Source: CAD feature listing. Evaluate the final solid. Frame: model axes, mm. A direction names the side the tool comes from. Coordinates: 2 decimals unless noted, no trailing zeros. Write each loop counter-clockwise with the first axis right and the second up, starting at its lowest first coordinate (ties: lowest second). Pieces come first, ordered by that corner, then holes. Notation, with made-up numbers: M 39,-28.75 L 95,-28.75 A31 cw 95,9.25 Z; hole C -29.5,2 d9. An arc over 180 degrees is marked long. Write item = value, one per line. Start each with the question number.
1. Line query: line 1 along Z through (x, y) = (15, 0.65); line 2 along X through (y, z) = (5.75, 8.75); line 3 along Z through (x, y) = (1.75, 5). Output: solid intervals per line, ascending.
2. Access query for faces 1 (the face through (12.86, 5.03, 0.81)), 2 (the face through (0, 3, 6)). Directions: +Z, -Z, +X, -X, +Y, -Y. A direction counts if a zero-diameter tool reaches every point of the face in a straight line with its end or side. Return the directions, or none.
3. Section query B-B (x = 15). Output: boundary loops of the cut face in (y, z), then the cut area to 3 significant figures.
4. Pin query (flat end, axial travel): pin 1 Ø0.9 at (x, z) = (1.5, 6) entering from +Y; pin 2 Ø2.5 at (x, z) = (1.5, 6) entering from +Y. Return the tip coordinate at first contact, or that it passes through.
5. Pull-direction query (Z, two-part tool) for faces 3 (the face through (10, 3, 0)), 4 (the face through (7.4, 1.6, 9.5)), 5 (the face through (19, 6.8, 9)); classes: pulls with the +Z half, pulls with the -Z half, needs draft (parallel to the pull), parting line crosses it, or undercut.
6. Section query A-A (y = 3.75). Output: boundary loops of the cut face in (x, z).
7. Section query C-C (z = 9). Output: boundary loops of the cut face in (x, y), then the cut area to 3 significant figures.
8. Section query D-D (x = 12.75). Output: boundary loops of the cut face in (y, z).
```python
from build123d import *

# Parameters (mm, degrees)
SKETCH_1_W          = 20
SKETCH_1_H          = 12
SKETCH_1_R          = 2.1
SKETCH_1_R_2        = 0.6
EXTRUDE_1_DEPTH     = 3.3
EXTRUDE_START       = 3.3
EXTRUDE_4_DEPTH     = 3.5
SKETCH_2_R          = 0.75
CUT_EXTRUDE_1_DEPTH = 29.930952283
CUT_EXTRUDE_START   = 24
SKETCH_2_4_R        = 1
CUT_EXTRUDE_2_DEPTH = 5.8
SKETCH_3_R          = 0.35
CUT_EXTRUDE_3_DEPTH = 25.294855422


with BuildPart() as part:
    # 草图1 → 凸台-拉伸1 (new body)
    with BuildSketch(Plane(origin=(0, 0, 0), x_dir=(1, 0, 0), z_dir=(0, 1, 0))):
        with Locations((10, -6)):
            Rectangle(SKETCH_1_W, SKETCH_1_H)
        with BuildLine():
            ThreePointArc((12.439835428, -3.613463312), (18.220575086, -7.370363498), (11.50515478, -5.81011348))
            ThreePointArc((11.50515478, -5.81011348), (7.454652656, -2.789434091), (12.439835428, -3.613463312))
        make_face(mode=Mode.SUBTRACT)
        with Locations(Location((5, -6, 0), (0, 0, 270))):
            Circle(SKETCH_1_R, mode=Mode.SUBTRACT)
        with Locations(Location((7.678736094, -8.970584613, 0), (0, 0, 270))):
            Circle(SKETCH_1_R_2, mode=Mode.SUBTRACT)
    extrude(amount=EXTRUDE_1_DEPTH)

    # 草图1<6> → 凸台-拉伸4 (add)
    with BuildSketch(Plane(origin=(0, 0, 0), x_dir=(1, 0, 0), z_dir=(0, 1, 0)).offset(EXTRUDE_START)):
        with BuildLine():
            Line((7.958677072, 0), (0, 0))
            Line((0, 0), (0, -12))
            Line((0, -12), (5.925840657, -12))
            ThreePointArc((5.925840657, -12), (4.429268792, -10.270954659), (4.319841502, -7.986802561))
            ThreePointArc((4.319841502, -7.986802561), (3.000111311, -5.359340003), (5.600909971, -3.987810345))
            ThreePointArc((5.600909971, -3.987810345), (6.188678117, -1.644412009), (7.958677072, 0))
        make_face()
        with BuildLine():
            Line((20, 0), (11.735482653, 0))
            ThreePointArc((11.735482653, 0), (12.869036074, -0.819060885), (13.675372646, -1.961700559))
            ThreePointArc((13.675372646, -1.961700559), (18.910698319, -7.664012819), (11.171707216, -7.845717845))
            ThreePointArc((11.171707216, -7.845717845), (11.090844977, -7.871351024), (11.009487245, -7.895365208))
            ThreePointArc((11.009487245, -7.895365208), (10.945672327, -10.226422042), (9.43163153, -12))
            Line((9.43163153, -12), (20, -12))
            Line((20, -12), (20, 0))
        make_face()
    extrude(amount=EXTRUDE_4_DEPTH)

    # 草图2 → 切除-拉伸1 (cut, through all)
    with BuildSketch(Plane(origin=(5, -17.2, 6), x_dir=(0, 0, -1), z_dir=(0, 1, 0))):
        with Locations(Location((0, 3.5, 0), (0, 0, 180))):
            Circle(SKETCH_2_R)
        with Locations(Location((-4.7, -10, 0), (0, 0, 49.37814182))):
            Circle(SKETCH_2_R)
        with Locations(Location((4.7, -10, 0), (0, 0, 229.37814182))):
            Circle(SKETCH_2_R)
    extrude(amount=CUT_EXTRUDE_1_DEPTH, mode=Mode.SUBTRACT)

    # 草图2<4> → 切除-拉伸2 (cut)
    with BuildSketch(Plane(origin=(5, -17.2, 6), x_dir=(0, 0, -1), z_dir=(0, 1, 0)).offset(CUT_EXTRUDE_START)):
        with Locations(Location((0, 3.5, 0), (0, 0, 180))):
            Circle(SKETCH_2_4_R)
        with Locations(Location((-4.7, -10, 0), (0, 0, 180))):
            Circle(SKETCH_2_4_R)
        with Locations(Location((4.7, -10, 0), (0, 0, 180))):
            Circle(SKETCH_2_4_R)
    extrude(amount=-CUT_EXTRUDE_2_DEPTH, mode=Mode.SUBTRACT)

    # 草图3 → 切除-拉伸3 (cut, through all)
    with BuildSketch(Plane(origin=(0, 0, 0), x_dir=(1, 0, 0), z_dir=(0, 1, 0))):
        with Locations(Location((1.5, -1.5, 0), (0, 0, 270))):
            Circle(SKETCH_3_R)
        with Locations(Location((1.5, -10.5, 0), (0, 0, 270))):
            Circle(SKETCH_3_R)
        with Locations(Location((18.5, -10.5, 0), (0, 0, 270))):
            Circle(SKETCH_3_R)
        with Locations(Location((18.5, -1.5, 0), (0, 0, 270))):
            Circle(SKETCH_3_R)
    extrude(amount=CUT_EXTRUDE_3_DEPTH, mode=Mode.SUBTRACT)


solid = part.part
```
Results are:
q1.line_1 = 0 to 0.55, 2.05 to 2.5, 9.5 to 9.95, 11.45 to 12
q1.line_2 = 0 to 4.19, 11.17 to 11.76, 18.24 to 20
q1.line_3 = 0 to 1.26, 1.74 to 5.03, 6.97 to 10.26, 10.74 to 12
q2.face_1 = +Y
q2.face_2 = +Z, -Z, -X, +Y, -Y
q3.outline = M 0,0 L 6.8,0 L 6.8,0.3 L 1,0.3 L 1,0.55 L 0,0.55 Z; M 0,2.05 L 1,2.05 L 1,2.3 L 3.3,2.3 L 3.3,2.5 L 0,2.5 Z; M 0,9.5 L 3.3,9.5 L 3.3,9.7 L 1,9.7 L 1,9.95 L 0,9.95 Z; M 0,11.45 L 1,11.45 L 1,11.7 L 6.8,11.7 L 6.8,12 L 0,12 Z
q3.area = 6.40 mm^2
q4.pin_1 = through
q4.pin_2 = 6.8
q5.face_3 = pulls with the -Z half
q5.face_4 = undercut
q5.face_5 = needs draft
q6.outline = M 0,0 L 7.96,0 A4.25 cw 5.6,3.99 A2.1 cw 4.32,7.99 A3.5 cw 5.93,12 L 0,12 Z; M 9.43,12 A3.5 cw 11.01,7.9 A4.25 cw 11.17,7.85 A4.25 cw 14.16,10.17 A1 cw long 15.84,10.17 A4.25 cw 15.84,1.83 A1 cw long 14.16,1.83 A4.25 cw 13.68,1.96 A4.25 cw 11.74,0 L 20,0 L 20,12 Z; hole C 1.5,6 d2; hole C 1.5,1.5 d0.7; hole C 1.5,10.5 d0.7; hole C 18.5,1.5 d0.7; hole C 18.5,10.5 d0.7
q7.outline = M 0,0 L 7.08,0 L 7.08,3.3 L 4.18,3.3 L 4.18,6.8 L 0,6.8 Z; M 8.28,0 L 13.2,0 L 13.2,3.3 L 11.99,3.3 L 11.99,6.8 L 11.18,6.8 L 11.18,3.3 L 8.28,3.3 Z; M 16.8,0 L 20,0 L 20,6.8 L 18.01,6.8 L 18.01,3.3 L 16.8,3.3 Z
q7.area = 74.6 mm^2
q8.outline = M 0,0 L 6.8,0 L 6.8,0.7 L 3.3,0.7 L 3.3,3.32 L 0,3.32 Z; M 0,8.68 L 3.3,8.68 L 3.3,9.61 L 6.8,9.61 L 6.8,12 L 0,12 Z
